from build123d import *

# Parameters (mm, degrees)
CHAMFER1_SIZE       = 0.35
CHAMFER1_SIZE2      = 1.306217783
CHAMFER2_SIZE       = 0.35
CHAMFER2_SIZE2      = 1.306217783
BOSS_EXTRUDE1_DEPTH = 7.4
SKETCH6_R           = 1.5
CUT_EXTRUDE1_DEPTH  = 10
CIRPATTERN1_COUNT   = 2
CIRPATTERN1_ANGLE   = 270


with BuildPart() as part:
    # Sketch2 → Revolve1 (revolve)
    with BuildSketch(Plane(origin=(0, 0, 0), x_dir=(0, 0, -1), z_dir=(1, 0, 0))):
        Polygon((-16, 4), (0, 4), (0, 8.5), (-7.6, 8.5), (-7.6, 5.8), (-15, 5.8), (-15, 8.5), (-16, 8.5), align=None)
    revolve(axis=Axis((0, 0, 79.609460318), (0, 0, -1)))

    # Chamfer1
    chamfer1_edges = [part.edges().sort_by_distance(p)[0] for p in [
        (0, -8.5, 15),
    ]]
    chamfer1_side = [part.faces().sort_by_distance(p)[0] for p in [
        (0, -8.5, 15.5),
    ]]
    chamfer(chamfer1_edges, length=CHAMFER1_SIZE, length2=CHAMFER1_SIZE2, reference=chamfer1_side[0])

    # Chamfer2
    chamfer2_edges = [part.edges().sort_by_distance(p)[0] for p in [
        (0, -8.5, 7.6),
    ]]
    chamfer2_side = [part.faces().sort_by_distance(p)[0] for p in [
        (0, -8.5, 3.8),
    ]]
    chamfer(chamfer2_edges, length=CHAMFER2_SIZE, length2=CHAMFER2_SIZE2, reference=chamfer2_side[0])

    # Sketch4 → Boss-Extrude1 (add)
    with BuildSketch(Plane.XY.offset(7.6)):
        with BuildLine():
            Line((1.645655792, 5.873824735), (1.892869388, 6.634669948))
            Line((1.892869388, 6.634669948), (2.368397646, 6.48016145))
            Line((2.368397646, 6.48016145), (2.121184051, 5.719316237))
            ThreePointArc((2.121184051, 5.719316237), (1.885003666, 5.801444749), (1.645655792, 5.873824735))
        make_face()
        with BuildLine():
            Line((-0.25, 6.094874896), (-0.25, 6.894874896))
            Line((-0.25, 6.894874896), (0.25, 6.894874896))
            Line((0.25, 6.894874896), (0.25, 6.094874896))
            ThreePointArc((0.25, 6.094874896), (0, 6.1), (-0.25, 6.094874896))
        make_face()
        with BuildLine():
            Line((3.38022333, 5.077803683), (3.850451532, 5.725017278))
            Line((3.850451532, 5.725017278), (4.254960029, 5.431124652))
            Line((4.254960029, 5.431124652), (3.784731827, 4.783911057))
            ThreePointArc((3.784731827, 4.783911057), (3.585490039, 4.935003666), (3.38022333, 5.077803683))
        make_face()
        with BuildLine():
            Line((4.783911057, 3.784731827), (5.431124652, 4.254960029))
            Line((5.431124652, 4.254960029), (5.725017278, 3.850451532))
            Line((5.725017278, 3.850451532), (5.077803683, 3.38022333))
            ThreePointArc((5.077803683, 3.38022333), (4.935003666, 3.585490039), (4.783911057, 3.784731827))
        make_face()
        with BuildLine():
            Line((5.719316237, 2.121184051), (6.48016145, 2.368397646))
            Line((6.48016145, 2.368397646), (6.634669948, 1.892869388))
            Line((6.634669948, 1.892869388), (5.873824735, 1.645655792))
            ThreePointArc((5.873824735, 1.645655792), (5.801444749, 1.885003666), (5.719316237, 2.121184051))
        make_face()
        with BuildLine():
            Line((6.094874896, 0.25), (6.894874896, 0.25))
            Line((6.894874896, 0.25), (6.894874896, -0.25))
            Line((6.894874896, -0.25), (6.094874896, -0.25))
            ThreePointArc((6.094874896, -0.25), (6.1, 0), (6.094874896, 0.25))
        make_face()
        with BuildLine():
            Line((5.873824735, -1.645655792), (6.634669948, -1.892869388))
            Line((6.634669948, -1.892869388), (6.48016145, -2.368397646))
            Line((6.48016145, -2.368397646), (5.719316237, -2.121184051))
            ThreePointArc((5.719316237, -2.121184051), (5.801444749, -1.885003666), (5.873824735, -1.645655792))
        make_face()
        with BuildLine():
            Line((5.077803683, -3.38022333), (5.725017278, -3.850451532))
            Line((5.725017278, -3.850451532), (5.431124652, -4.254960029))
            Line((5.431124652, -4.254960029), (4.783911057, -3.784731827))
            ThreePointArc((4.783911057, -3.784731827), (4.935003666, -3.585490039), (5.077803683, -3.38022333))
        make_face()
        with BuildLine():
            Line((3.784731827, -4.783911057), (4.254960029, -5.431124652))
            Line((4.254960029, -5.431124652), (3.850451532, -5.725017278))
            Line((3.850451532, -5.725017278), (3.38022333, -5.077803683))
            ThreePointArc((3.38022333, -5.077803683), (3.585490039, -4.935003666), (3.784731827, -4.783911057))
        make_face()
        with BuildLine():
            Line((2.121184051, -5.719316237), (2.368397646, -6.48016145))
            Line((2.368397646, -6.48016145), (1.892869388, -6.634669948))
            Line((1.892869388, -6.634669948), (1.645655792, -5.873824735))
            ThreePointArc((1.645655792, -5.873824735), (1.885003666, -5.801444749), (2.121184051, -5.719316237))
        make_face()
        with BuildLine():
            Line((0.25, -6.094874896), (0.25, -6.894874896))
            Line((0.25, -6.894874896), (-0.25, -6.894874896))
            Line((-0.25, -6.894874896), (-0.25, -6.094874896))
            ThreePointArc((-0.25, -6.094874896), (0, -6.1), (0.25, -6.094874896))
        make_face()
        with BuildLine():
            Line((-1.645655792, -5.873824735), (-1.892869388, -6.634669948))
            Line((-1.892869388, -6.634669948), (-2.368397646, -6.48016145))
            Line((-2.368397646, -6.48016145), (-2.121184051, -5.719316237))
            ThreePointArc((-2.121184051, -5.719316237), (-1.885003666, -5.801444749), (-1.645655792, -5.873824735))
        make_face()
        with BuildLine():
            Line((-3.38022333, -5.077803683), (-3.850451532, -5.725017278))
            Line((-3.850451532, -5.725017278), (-4.254960029, -5.431124652))
            Line((-4.254960029, -5.431124652), (-3.784731827, -4.783911057))
            ThreePointArc((-3.784731827, -4.783911057), (-3.585490039, -4.935003666), (-3.38022333, -5.077803683))
        make_face()
        with BuildLine():
            Line((-4.783911057, -3.784731827), (-5.431124652, -4.254960029))
            Line((-5.431124652, -4.254960029), (-5.725017278, -3.850451532))
            Line((-5.725017278, -3.850451532), (-5.077803683, -3.38022333))
            ThreePointArc((-5.077803683, -3.38022333), (-4.935003666, -3.585490039), (-4.783911057, -3.784731827))
        make_face()
        with BuildLine():
            Line((-5.719316237, -2.121184051), (-6.48016145, -2.368397646))
            Line((-6.48016145, -2.368397646), (-6.634669948, -1.892869388))
            Line((-6.634669948, -1.892869388), (-5.873824735, -1.645655792))
            ThreePointArc((-5.873824735, -1.645655792), (-5.801444749, -1.885003666), (-5.719316237, -2.121184051))
        make_face()
        with BuildLine():
            Line((-6.094874896, -0.25), (-6.894874896, -0.25))
            Line((-6.894874896, -0.25), (-6.894874896, 0.25))
            Line((-6.894874896, 0.25), (-6.094874896, 0.25))
            ThreePointArc((-6.094874896, 0.25), (-6.1, 0), (-6.094874896, -0.25))
        make_face()
        with BuildLine():
            Line((-5.873824735, 1.645655792), (-6.634669948, 1.892869388))
            Line((-6.634669948, 1.892869388), (-6.48016145, 2.368397646))
            Line((-6.48016145, 2.368397646), (-5.719316237, 2.121184051))
            ThreePointArc((-5.719316237, 2.121184051), (-5.801444749, 1.885003666), (-5.873824735, 1.645655792))
        make_face()
        with BuildLine():
            Line((-5.077803683, 3.38022333), (-5.725017278, 3.850451532))
            Line((-5.725017278, 3.850451532), (-5.431124652, 4.254960029))
            Line((-5.431124652, 4.254960029), (-4.783911057, 3.784731827))
            ThreePointArc((-4.783911057, 3.784731827), (-4.935003666, 3.585490039), (-5.077803683, 3.38022333))
        make_face()
        with BuildLine():
            Line((-3.784731827, 4.783911057), (-4.254960029, 5.431124652))
            Line((-4.254960029, 5.431124652), (-3.850451532, 5.725017278))
            Line((-3.850451532, 5.725017278), (-3.38022333, 5.077803683))
            ThreePointArc((-3.38022333, 5.077803683), (-3.585490039, 4.935003666), (-3.784731827, 4.783911057))
        make_face()
        with BuildLine():
            Line((-2.121184051, 5.719316237), (-2.368397646, 6.48016145))
            Line((-2.368397646, 6.48016145), (-1.892869388, 6.634669948))
            Line((-1.892869388, 6.634669948), (-1.645655792, 5.873824735))
            ThreePointArc((-1.645655792, 5.873824735), (-1.885003666, 5.801444749), (-2.121184051, 5.719316237))
        make_face()
    extrude(amount=BOSS_EXTRUDE1_DEPTH)

    # Sketch6 → Cut-Extrude1 (cut)
    with BuildSketch(Plane(origin=(0, 8.9, 0), x_dir=(-1, 0, 0), z_dir=(0, 1, 0))):
        with Locations((0, 3.55)):
            Circle(SKETCH6_R)
    cut_extrude1 = extrude(amount=-CUT_EXTRUDE1_DEPTH, mode=Mode.SUBTRACT)

    # CirPattern1: Cut-Extrude1 ×2 about axis
    cirpattern1_axis = Axis((0, 0, 0), (0, 0, 1))
    for i in range(1, CIRPATTERN1_COUNT):
        add(cut_extrude1.rotate(cirpattern1_axis, i * CIRPATTERN1_ANGLE / (CIRPATTERN1_COUNT - 1)), mode=Mode.SUBTRACT)


solid = part.part
Source: CAD feature listing. Evaluate the final solid. Frame: model axes, mm. A direction names the side the tool comes from. Round coordinates to 2 decimals unless told otherwise and drop trailing zeros. Loops run counter-clockwise (first coordinate to the right, second up) from the corner with the lowest first, then second, coordinate; pieces in that order, holes last. Notation, with made-up numbers: M 5,-0.75 L 40,-0.75 A25 ccw 40,14.25 Z; hole C -10.5,84.5 d3. An arc over 180 degrees is marked long. Return JSON: item names as keys, results as strings. Group by question number.
1. Section query C-C on z = 3.55. Output: boundary loops of the cut face in (x, y), and give its area (3 significant figures).
2. Material intervals for line 1 along Y through (x, z) = (2, 14.5); line 2 along X through (y, z) = (0, 8); line 3 along X through (y, z) = (0, 5.75), sorted ascending. Write a range as from..to.
3. Mould query, pull axis X, two halves, no side actions, for faces 3 (the face through (6.139, -0.195, 5.037)), 4 (the face through (0.195, 6.138, 5.037)), 5 (the face through (7.167, 4.57, 15.68)). Classes: released by +X, released by -X, zero draft, split by the parting line, or undercut.
4. Pin query (flat end, axial travel): pin 1 (1.5 mm diameter, centred on y = -5, z = 3, fed in from +X); pin 2 (2.5 mm diameter, centred on x = 0, z = 3.55, fed in from +Y); pin 3 (0.6 mm diameter, centred on x = 6.5, z = 10.5, fed in from +Y). Return the tip coordinate at first contact, or that it passes through.
5. Reachability of faces 1 (the face through (6, -1, 7.6)), 2 (the face through (-2, 4, 16)) from +Z, -Z, +X, -X, +Y, -Y: full face, straight path, thin tool, end or side. Return the list, or none.
6. Section query A-A on y = 0. State how many separate pieces and enclosed holes the cut face has, and give its area (3 significant figures).
Checks:
{
 "1": {"outline": "M -1.5,3.71 L -1.5,8.37 A8.5 ccw long 8.37,-1.5 L 3.71,-1.5 A4 cw long Z; M 1.5,3.71 A4 cw 3.71,1.5 L 8.37,1.5 A8.5 ccw 1.5,8.37 Z", "area": "149 mm²"},
 "2": {"line 1": "y = -6.6..-5.76, -5.44..-3.46, 3.46..5.44, 5.76..6.6", "line 2": "x = -6.89..-6.1, -5.8..-4, 4..5.8, 6.1..6.89", "line 3": "x = -8.5..-4, 4..8.5"},
 "3": {"face 3": "zero draft", "face 4": "undercut", "face 5": "split by the parting line"},
 "4": {"pin 1": "stops at x = 7.36", "pin 2": "stops at y = -3.8", "pin 3": "stops at y = 2.37"},
 "5": {"face 1": "none", "face 2": "+Z, +X, -X, +Y, -Y"},
 "6": {"separate pieces": "3", "enclosed holes": "2", "area": "101 mm²"}
}
